The model under review builds one solid part; all positions refer to its coordinate system, in mm. Face numbers are marked on the shaded views. A direction names the side the tool comes from. Coordinates: 2 decimals unless noted, no trailing zeros. Write each loop counter-clockwise with the first axis right and the second up, starting at its lowest first coordinate (ties: lowest second). Pieces come first, ordered by that corner, then holes. Notation, with made-up numbers: (23.5, 33) -> (43.5, 33) arc R19 cw to (43.5, 65) -> close; hole circle Ø6 at (49.25, 24.25). An arc over 180 degrees is marked (long way). Write each question's results on one line, items separated by ' | '.
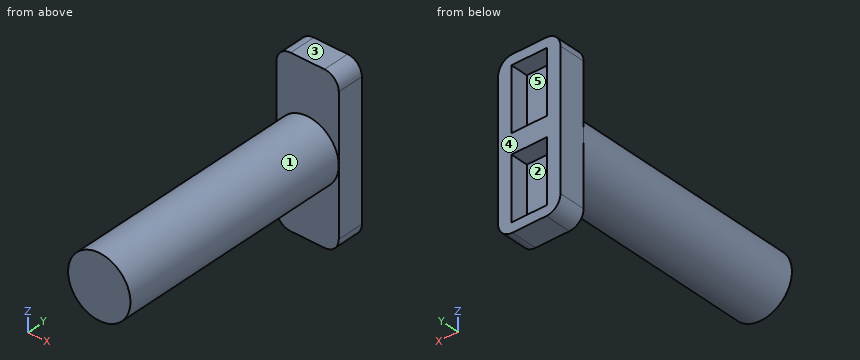
```python
from build123d import *

# Parameters (mm, degrees)
SKETCH1_R           = 17.5
BOSS_EXTRUDE1_DEPTH = 150
SKETCH2_W           = 35
SKETCH2_H           = 15
BOSS_EXTRUDE2_DEPTH = 46
SKETCH3_W           = 20
SKETCH3_H           = 35
CUT_EXTRUDE1_DEPTH  = 10
FILLET1_R           = 8


with BuildPart() as part:
    # Sketch1 → Boss-Extrude1 (new body)
    with BuildSketch(Plane(origin=(0, 0, 0), x_dir=(1, 0, 0), z_dir=(0, 1, 0))):
        with Locations(Location((0, 0, 0), (0, 0, 270))):
            Circle(SKETCH1_R)
    extrude(amount=BOSS_EXTRUDE1_DEPTH)

    # Sketch2 → Boss-Extrude2 (add, symmetric)
    with BuildSketch(Plane.XY):
        with Locations((0, 142.5)):
            Rectangle(SKETCH2_W, SKETCH2_H)
    extrude(amount=BOSS_EXTRUDE2_DEPTH, both=True)

    # Sketch3 → Cut-Extrude1 (cut)
    with BuildSketch(Plane(origin=(0, 150, 0), x_dir=(1, 0, 0), z_dir=(0, 1, 0))):
        with Locations((0, 23)):
            Rectangle(SKETCH3_W, SKETCH3_H)
        with Locations((0, -23)):
            Rectangle(SKETCH3_W, SKETCH3_H)
    extrude(amount=-CUT_EXTRUDE1_DEPTH, mode=Mode.SUBTRACT)

    # Fillet1
    fillet1_edges = [part.edges().sort_by_distance(p)[0] for p in [
        (-17.5, 142.5, 46),
        (17.5, 142.5, 46),
        (17.5, 142.5, -46),
        (-17.5, 142.5, -46),
    ]]
    fillet(fillet1_edges, radius=FILLET1_R)


solid = part.part
```
Q1. Clearance check with flat-ended pins moving along their axes: P1, Ø2, axis at x = 1, y = 68.5, coming from the +Z side; P2, Ø10, axis at x = 3, z = 24, coming from the +Y side; P3, Ø2, axis at y = 39.5, z = -13, coming from the +X side. State where each tip first meets the part, or that it passes through.
Solution:
P1: z = 17.5 | P2: y = 140 | P3: x = 12.74
Q2. Add section A-A (z = 36.5). Write out the cut boundary in (x, y), plus the area to 3 significant figures.
Solution:
outline: (-17.5, 135) -> (17.5, 135) -> (17.5, 150) -> (10, 150) -> (10, 140) -> (-10, 140) -> (-10, 150) -> (-17.5, 150) -> close | area: 325 mm²
Q3. Add section C-C (y = 37.5). Write out the cut boundary in (x, z).
Solution:
outline: circle Ø35 at (0, 0)
Q4. Draft analysis for pull direction X (two halves, no side actions). For the marked faces 1, 2 and 3, state which applies: pulls with the +X half, pulls with the -X half, needs draft (parallel to the pull), parting line crosses it, or undercut.
Solution:
face 1: parting line crosses it | face 2: undercut | face 3: needs draft
Q5. Add section B-B (x = 0). Write out the cut boundary in (y, z), plus the area to 4 significant figures.
Solution:
outline: (0, -17.5) -> (135, -17.5) -> (135, -46) -> (150, -46) -> (150, -40.5) -> (140, -40.5) -> (140, -5.5) -> (150, -5.5) -> (150, 5.5) -> (140, 5.5) -> (140, 40.5) -> (150, 40.5) -> (150, 46) -> (135, 46) -> (135, 17.5) -> (0, 17.5) -> close | area: 5,405 mm²
Q6. For line 1 (Y direction, x = -3.5, z = 28.5); line 2 (Y direction, x = 13, z = -41.5); line 3 (Z direction, x = 0.5, y = 14.5), list the stretches that pass through material, from the lowest coordinate up. Write a range as from..to.
Solution:
line 1: 135..140 | line 2: 135..150 | line 3: -17.49..17.49
Q7. Machinability: for the marked faces 4 and 5, which of the approach directions +Z, -Z, +X, -X, +Y, -Y give a long, thin tool a straight path to every point of the face, cutting with its end or side? Answer none if there is none.
Solution:
face 4: +Z, -Z, +X, -X, +Y | face 5: +Y
Q8. Add section D-D (z = 12). Write out the cut boundary in (x, y), plus the area to 3 significant figures.
Solution:
outline: (-17.5, 135) -> (-12.74, 135) -> (-12.74, 0) -> (12.74, 0) -> (12.74, 135) -> (17.5, 135) -> (17.5, 150) -> (10, 150) -> (10, 140) -> (-10, 140) -> (-10, 150) -> (-17.5, 150) -> close | area: 3,760 mm²
